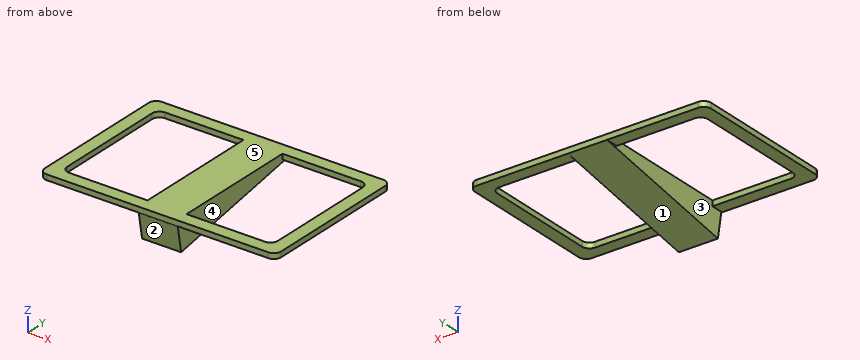
from build123d import *

# Parameters (mm, degrees)
PAD_DEPTH    = 5
PAD001_DEPTH = 18.25


with BuildPart() as part:
    # Sketch → Pad (new body)
    with BuildSketch(Plane.XY):
        with BuildLine():
            Line((7, 0), (214, 0))
            ThreePointArc((221, -7), (218.949747, -2.050253), (214, 0))
            Line((221, -7), (221, -137))
            ThreePointArc((214, -144), (218.949747, -141.949747), (221, -137))
            Line((214, -144), (7, -144))
            ThreePointArc((0, -137), (2.050253, -141.949747), (7, -144))
            Line((0, -137), (0, -7))
            ThreePointArc((7, 0), (2.050253, -2.050253), (0, -7))
        make_face()
        with BuildLine():
            Line((19, -12), (202, -12))
            ThreePointArc((209, -19), (206.949747, -14.050253), (202, -12))
            Line((209, -19), (209, -125))
            ThreePointArc((202, -132), (206.949747, -129.949747), (209, -125))
            Line((202, -132), (19, -132))
            ThreePointArc((12, -125), (14.050253, -129.949747), (19, -132))
            Line((12, -125), (12, -19))
            ThreePointArc((19, -12), (14.050253, -14.050253), (12, -19))
        make_face(mode=Mode.SUBTRACT)
    extrude(amount=PAD_DEPTH)

    # Sketch001 (on DatumPlane) → Pad001 (join, symmetric)
    with BuildSketch(Plane.YZ.offset(110.5)):
        Polygon((0, 0), (-138.802818, -24.474682), (-144, 5), (0, 5), align=None)
    extrude(amount=PAD001_DEPTH, both=True)


solid = part.part
Work out the finished part from the listing and answer in its coordinate system (mm). Face numbers are marked on the shaded views. A direction names the side the tool comes from. Round coordinates to 2 decimals unless told otherwise and drop trailing zeros. Order: outer loops, then holes, each group sorted by start corner. A loop starts at its lowest first (then second) coordinate and runs counter-clockwise, first axis right, second up. Notation, with made-up numbers: M 31.25,35 L 48.25,35 A18 ccw 48.25,39 Z; hole C 52,71.5 d11. An arc over 180 degrees is marked long. Put each result on its own line as item: value. Start each with the question number.
Q1. Section B-B, the plane y = -119.5 is taken. Write down the section's boundary in (x, z).
Q2. Section C-C, the plane x = 14.5 is taken. Write down the section's boundary in (y, z), and give its area (3 significant figures).
Q3. Section D-D, the plane z = -12.5 is taken. Write down the section's boundary in (x, y).
Q4. Straight lines are drawn through the part: L1, parallel to X at y = -124, z = 1.25; L2, parallel to Y at x = 64, z = 1.5; L3, parallel to X at y = -114.5, z = -19.75. For each, find the intervals that lie inside material, in ascending order. Write a range as [from, to].
Q5. For a pull along Y with two mould halves and no side action, classify the marked faces 1, 2 and 3 as pulls with the +Y half, pulls with the -Y half, needs draft (parallel to the pull), parting line crosses it, or undercut.
Q6. Section A-A, the plane x = 198 is taken. Write down the section's boundary in (y, z), and give its area (3 significant figures).
Q7. A tool of negligible diameter and unlimited length cuts with its end or side. For the marked faces 4 and 5, from which of +Z, -Z, +X, -X, +Y, -Y can it reach the whole face along a straight path? Write none if from no direction.
Q8. Flat-ended cylindrical pins translate along their axes: pin 1 (5.5 mm diameter, centred on x = 42, z = 2.5, fed in from +Y); pin 2 (3 mm diameter, centred on y = -79, z = -14, fed in from -X); pin 3 (1 mm diameter, centred on y = -80, z = -3, fed in from +X). Find the tip coordinate at first contact, or state that the pin passes through.
Findings below:
1. outline: M 0,0 L 12,0 L 12,5 L 0,5 Z; M 92.25,-21.07 L 128.75,-21.07 L 128.75,5 L 92.25,5 Z; M 209,0 L 221,0 L 221,5 L 209,5 Z
2. outline: M -144,0 L -130.36,0 L -130.36,5 L -144,5 Z; M -13.64,0 L 0,0 L 0,5 L -13.64,5 Z
2. area: 136 mm^2
3. outline: M 92.25,-140.91 L 128.75,-140.91 L 128.75,-70.89 L 92.25,-70.89 Z
4. L1: x = [0, 12], [92.25, 128.75], [209, 221]
4. L2: y = [-144, -132], [-12, 0]
4. L3: x = [92.25, 128.75]
5. face 1: pulls with the +Y half
5. face 2: pulls with the -Y half
5. face 3: undercut
6. outline: M -144,0 L -132,0 L -132,5 L -144,5 Z; M -12,0 L 0,0 L 0,5 L -12,5 Z
6. area: 120 mm^2
7. face 4: -Z
7. face 5: +Z, +X, -X, +Y, -Y
8. pin 1: stops at y = 0
8. pin 2: stops at x = 92.25
8. pin 3: stops at x = 128.75
